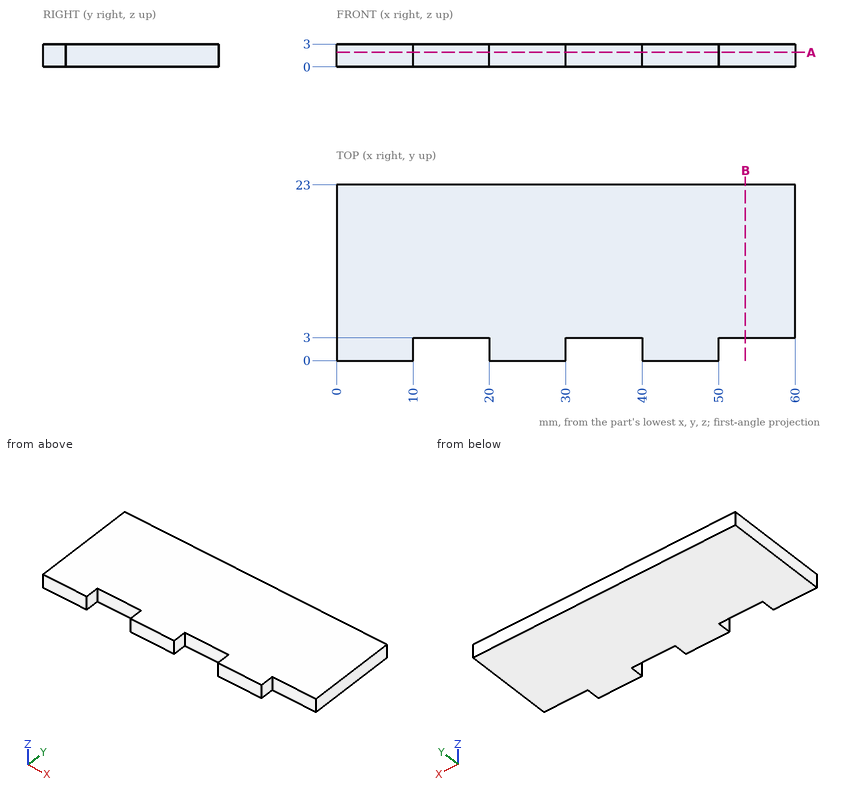
Design review of the part shown in the three views and the two pictorial views. Dimensions are in mm from the part's minimum x, y and z. Round coordinates to 2 decimals unless told otherwise and drop trailing zeros. Loops run counter-clockwise (first coordinate to the right, second up) from the corner with the lowest first, then second, coordinate; pieces in that order, holes last. Notation, with made-up numbers: (47.25, -38.5) - (73.25, -38.5) arc R10 ccw to (73.25, -19.5) - close; hole circle Ø9 at (0, 13). An arc over 180 degrees is marked (long way). One line per item, written item: value. Start each with the question number.
Item 1: Take a section at A-A (z = 1.9). Give the boundary of the cut face in (x, y).
Item 2: For L1, parallel to X at y = 1.5, z = 1.75; L2, parallel to Y at x = 55.5, z = 2.2, list the stretches that pass through material, from the lowest coordinate up.
Item 3: Clearance check with a flat-ended pin moving along its axis: pin 1 Ø1.5 at (x, z) = (36, 1.5) entering from -Y. State where the tip first meets the part, or that it passes through.
Item 4: Take a section at B-B (x = 53.5). Give the boundary of the cut face in (y, z).
Answer below:
1. outline: (0, 0) - (10, 0) - (10, 3) - (20, 3) - (20, 0) - (30, 0) - (30, 3) - (40, 3) - (40, 0) - (50, 0) - (50, 3) - (60, 3) - (60, 23) - (0, 23) - close
2. L1: x = 0 to 10, 20 to 30, 40 to 50
2. L2: y = 3 to 23
3. pin 1: stops at y = 3
4. outline: (3, 0) - (23, 0) - (23, 3) - (3, 3) - close
